```python
from build123d import *

# Parameters (mm, degrees)
F0_W     = 17.6849197596
F0_H     = 5.9900539927
F1_DEPTH = 25.4
F2_DEPTH = 29.92783
F3_DEPTH = 0.33087


with BuildPart() as f1:
    # F0 (on Front) → F1 (new body)
    with BuildSketch(Plane.XZ):
        Polygon((-27.0978603512, 4.4212299399), (-44.7827801108, 4.4212299399), (-49.9171130359, 4.4212299399), (-49.9171130359, -2.7097861748), (35.6550812721, -2.7097861748), (35.6550812721, 4.4212299399), align=None)
        Polygon((15.317424354, 11.6948666982), (14.7060211414, 16.9097762866), (-18.8258830458, 12.9784494638), (-20.2520862222, 11.6948666982), align=None)
        with Locations((-35.940320231, 7.4162569363)):
            Rectangle(F0_W, F0_H)
        Polygon((17.3996798694, 25.529038161), (-45.3532636166, 21.5356685221), (-49.9171130359, 14.11941275), (-49.9171130359, 10.4112839326), (-44.7827801108, 10.4112839326), (-27.0978603512, 10.4112839326), (-21.6782893986, 10.4112839326), (-20.2520862222, 11.6948666982), (-18.8258830458, 12.9784494638), (14.7060211414, 16.9097762866), (22.5340109318, 17.8275406361), align=None)
    extrude(amount=F1_DEPTH)

    # F0 (on Front) → F2 (join)
    with BuildSketch(Plane.XZ):
        Polygon((17.3996798694, 25.529038161), (-45.3532636166, 21.5356685221), (-49.9171130359, 14.11941275), (-49.9171130359, 10.4112839326), (-44.7827801108, 10.4112839326), (-27.0978603512, 10.4112839326), (-21.6782893986, 10.4112839326), (-20.2520862222, 11.6948666982), (-18.8258830458, 12.9784494638), (14.7060211414, 16.9097762866), (22.5340109318, 17.8275406361), align=None)
        Polygon((-27.0978603512, 4.4212299399), (-44.7827801108, 4.4212299399), (-49.9171130359, 4.4212299399), (-49.9171130359, -2.7097861748), (35.6550812721, -2.7097861748), (35.6550812721, 4.4212299399), align=None)
    extrude(amount=F2_DEPTH)

    # F3 (add): faces of the model
    f3_faces = [f1.faces().sort_by_distance(p)[0] for p in [
        (1.3459851792, -25.4, 13.5050170467),
        (-35.940320231, -25.4, 7.4162569363),
    ]]
    extrude(f3_faces, amount=F3_DEPTH)


solid = f1.part
```
Read the model definition and answer for the solid it produces. Units are mm, in the model's axes. A direction names the side the tool comes from. Round coordinates to 2 decimals unless told otherwise and drop trailing zeros. Write each loop counter-clockwise with the first axis right and the second up, starting at its lowest first coordinate (ties: lowest second). Pieces come first, ordered by that corner, then holes. Notation, with made-up numbers: (-9, 21.5) -> (20, 21.5) arc R27 cw to (20, 60.5) -> close; hole circle Ø4 at (85.5, 51). An arc over 180 degrees is marked (long way). Answer in a Markdown table with one row per item. Add a question column.
1) Which of the six approach directions +Z, -Z, +X, -X, +Y, -Y give full straight-line access (tool end or side, diameter ignored) to faces 1 (the face through (1, -25.731, 14)), 2 (the face through (-26.6, -14.8, 10.411)), 3 (the face through (-44.783, -13, 7)), 4 (the face through (-47.603, -14.754, 17.879)), 5 (the face through (-3, -13, 11.695))?
2) Find section D-D, the plane z = 7. Determine the outline of the cut face in (x, y), and give its area (3 significant figures).
3) Consider line 1 (Z direction, x = 24, y = -24); line 2 (Y direction, x = -37.5, z = 5.5); line 3 (X direction, y = -11.75, z = 7.5). Determine where each line is inside the solid, lowest interval first.
4) Given P1, Ø3, axis at y = -17, z = 7.5, coming from the +X side; P2, Ø2, axis at y = -18, z = 8, coming from the -X side; P3, Ø2, axis at y = -6.5, z = 17, coming from the +X side, each flat-ended and moving along its own axis, determine where each tip first touches the part or whether it passes through.
5) Find section B-B, the plane y = -21.5. Determine the outline of the cut face in (x, z).
6) Find section A-A, the plane x = 12.5. Determine the outline of the cut face in (y, z).
7) Determine the mould class of faces 6 (the face through (20.003, -14.754, 21.624)), 7 (the face through (3, -15, 4.421)), 8 (the face through (-36, -25.731, 7)), 9 (the face through (-8, -29.928, 1)) for opening direction Z: pulls with the +Z half, pulls with the -Z half, needs draft (parallel to the pull), parting line crosses it, or undercut.
8) Find section C-C, the plane x = -38. Determine the outline of the cut face in (y, z), and give its area (3 significant figures).
Findings below:
| question | item | result |
|---|---|---|
| 1 | face 1 | +X, -Y |
| 1 | face 2 | -Y |
| 1 | face 3 | -X, +Y, -Y |
| 1 | face 4 | +Z, -X, +Y, -Y |
| 1 | face 5 | +X, +Y, -Y |
| 2 | outline | (-44.78, -25.73) -> (-27.1, -25.73) -> (-27.1, 0) -> (-44.78, 0) -> close |
| 2 | area | 455 mm² |
| 3 | line 1 | -2.71 to 4.42 |
| 3 | line 2 | -25.73 to 0 |
| 3 | line 3 | -44.78 to -27.1 |
| 4 | P1 | x = -27.1 |
| 4 | P2 | x = -44.78 |
| 4 | P3 | x = 22.53 |
| 5 | outline | (-49.92, -2.71) -> (35.66, -2.71) -> (35.66, 4.42) -> (-27.1, 4.42) -> (-27.1, 10.41) -> (-21.68, 10.41) -> (-20.25, 11.69) -> (15.32, 11.69) -> (14.71, 16.91) -> (22.53, 17.83) -> (17.4, 25.53) -> (-45.35, 21.54) -> (-49.92, 14.12) -> (-49.92, 10.41) -> (-44.78, 10.41) -> (-44.78, 4.42) -> (-49.92, 4.42) -> close |
| 6 | outline | (-29.93, -2.71) -> (0, -2.71) -> (0, 4.42) -> (-29.93, 4.42) -> close; (-29.93, 16.65) -> (-25.73, 16.65) -> (-25.73, 11.69) -> (0, 11.69) -> (0, 25.22) -> (-29.93, 25.22) -> close |
| 7 | face 6 | pulls with the +Z half |
| 7 | face 7 | undercut |
| 7 | face 8 | undercut |
| 7 | face 9 | needs draft |
| 8 | outline | (-29.93, -2.71) -> (0, -2.71) -> (0, 22) -> (-29.93, 22) -> (-29.93, 10.41) -> (-25.73, 10.41) -> (-25.73, 4.42) -> (-29.93, 4.42) -> close |
| 8 | area | 714 mm² |
